Geometry: final body of the model. Coordinates: model frame, mm. A direction names the side the tool comes from. Coordinates: 2 decimals unless noted, no trailing zeros. Order: outer loops, then holes, each group sorted by start corner. A loop starts at its lowest first (then second) coordinate and runs counter-clockwise, first axis right, second up. Notation, with made-up numbers: M -21.5,84 L 32.5,84 A27 cw 32.5,108 Z; hole C -39.5,89 d9. An arc over 180 degrees is marked long. Use CSV: the item, a comma, the result in double quotes. Start each with the question number.
Q1. First-contact query: P1, Ø1, axis at x = 8.5, y = 3.5, coming from the -Z side; P2, Ø1.2, axis at x = 13.5, z = 4, coming from the -Y side; P3, Ø4, axis at x = -3.5, z = 4, coming from the -Y side. Flat tips, straight axial feed; report the tip coordinate or a pass-through.
Q2. Section query D-D, the plane z = 6.25. Output: boundary loops of the cut face in (x, y).
Q3. Mould query, pull axis X, two halves, no side actions, for faces 1 (the face through (16.25, -3, 4)), 2 (the face through (-16.25, -3, 4)), 3 (the face through (13, -1, 4)), 4 (the face through (-14, -11, 5)). Classes: +X half, -X half, draft (parallel to the pull), parting line (faces both ways), or undercut.
Q4. Section query A-A, the plane y = -9.25. Output: boundary loops of the cut face in (x, z), and give its area (3 significant figures).
Q5. Section query B-B, the plane z = 4. Output: boundary loops of the cut face in (x, y), and give its area (4 significant figures).
Q6. Ray query, probe 1 along Z at (x, y) = (13.5, -6.25); probe 2 along X at (y, z) = (-8, 2.75); probe 3 along Y at (x, z) = (10.5, 3). Return the intervals inside material, ascending.
Q7. Access query for faces 5 (the face through (0, 5, 4)), 6 (the face through (11.25, -5, 4)), 7 (the face through (-14, -1, 4)). Directions: +Z, -Z, +X, -X, +Y, -Y. A direction counts if a zero-diameter tool reaches every point of the face in a straight line with its end or side. Return the directions, or none.
Q8. Section query C-C, the plane x = -13.5. Output: boundary loops of the cut face in (y, z), and give its area (3 significant figures).
from build123d import *

# Parameters (mm, degrees)
PAD_DEPTH    = 8
SKETCH001_R  = 0.75
POCKET_DEPTH = 10


with BuildPart() as part:
    # Sketch → Pad (new body)
    with BuildSketch(Plane.XY):
        Polygon((11.25, 0), (11.25, -11), (16.25, -11), (16.25, 5), (-16.25, 5), (-16.25, -11), (-11.25, -11), (-11.25, 0), align=None)
    extrude(amount=PAD_DEPTH)

    # Sketch001 (on Face6 of Pad) → Pocket (cut)
    with BuildSketch(Plane.XZ.offset(11)):
        with Locations((-13.5, 4)):
            Circle(SKETCH001_R)
        with Locations((13.5, 4)):
            Circle(SKETCH001_R)
    extrude(amount=-POCKET_DEPTH, mode=Mode.SUBTRACT)


solid = part.part
Responses:
1,P1,"stops at z = 0"
1,P2,"stops at y = -1"
1,P3,"stops at y = 0"
2,outline,"M -16.25,-11 L -11.25,-11 L -11.25,0 L 11.25,0 L 11.25,-11 L 16.25,-11 L 16.25,5 L -16.25,5 Z"
3,face 1,"+X half"
3,face 2,"-X half"
3,face 3,"undercut"
3,face 4,"draft"
4,outline,"M -16.25,0 L -11.25,0 L -11.25,8 L -16.25,8 Z; M 11.25,0 L 16.25,0 L 16.25,8 L 11.25,8 Z; hole C -13.5,4 d1.5; hole C 13.5,4 d1.5"
4,area,"76.5 mm²"
5,outline,"M -16.25,-11 L -14.25,-11 L -14.25,-1 L -12.75,-1 L -12.75,-11 L -11.25,-11 L -11.25,0 L 11.25,0 L 11.25,-11 L 12.75,-11 L 12.75,-1 L 14.25,-1 L 14.25,-11 L 16.25,-11 L 16.25,5 L -16.25,5 Z"
5,area,"242.5 mm²"
6,probe 1,"z = 0 to 3.25, 4.75 to 8"
6,probe 2,"x = -16.25 to -11.25, 11.25 to 16.25"
6,probe 3,"y = 0 to 5"
7,face 5,"+Z, -Z, +X, -X, +Y"
7,face 6,"+Z, -Z, -Y"
7,face 7,"-Y"
8,outline,"M -11,0 L 5,0 L 5,8 L -11,8 L -11,4.75 L -1,4.75 L -1,3.25 L -11,3.25 Z"
8,area,"113 mm²"
